```python
from build123d import *

# Parameters (mm, degrees)
SKETCH1_R           = 16.25
BOSS_EXTRUDE1_DEPTH = 84
SKETCH2_R           = 10
BOSS_EXTRUDE2_DEPTH = 3
SKETCH3_R           = 3
BOSS_EXTRUDE3_DEPTH = 17
CUT_EXTRUDE1_DEPTH  = 12
SKETCH5_R           = 16.25
BOSS_EXTRUDE4_DEPTH = 18
SKETCH6_W           = 8.15482979
SKETCH6_H           = 20.288083416
BOSS_EXTRUDE5_DEPTH = 16


with BuildPart() as part:
    # Sketch1 → Boss-Extrude1 (new body)
    with BuildSketch(Plane(origin=(0, 0, 0), x_dir=(0, 0, -1), z_dir=(1, 0, 0))):
        Circle(SKETCH1_R)
    extrude(amount=BOSS_EXTRUDE1_DEPTH)

    # Sketch2 → Boss-Extrude2 (add)
    with BuildSketch(Plane(origin=(84, 0, 0), x_dir=(0, 0, -1), z_dir=(1, 0, 0))):
        Circle(SKETCH2_R)
    extrude(amount=BOSS_EXTRUDE2_DEPTH)

    # Sketch3 → Boss-Extrude3 (add)
    with BuildSketch(Plane(origin=(87, 0, 0), x_dir=(0, 0, -1), z_dir=(1, 0, 0))):
        Circle(SKETCH3_R)
    extrude(amount=BOSS_EXTRUDE3_DEPTH)

    # Sketch4 → Cut-Extrude1 (cut)
    with BuildSketch(Plane(origin=(104, 0, 0), x_dir=(0, 0, -1), z_dir=(1, 0, 0))):
        Polygon((-63.514658307, 2.5), (-1.658312395, 2.5), (1.658312395, 2.5), (63.514658307, 2.5), (63.514658307, 126.212691825), (-63.514658307, 126.212691825), align=None)
    extrude(amount=-CUT_EXTRUDE1_DEPTH, mode=Mode.SUBTRACT)

    # Sketch5 → Boss-Extrude4 (add)
    with BuildSketch(Plane.ZY):
        Circle(SKETCH5_R)
        with BuildLine():
            Line((-16.25, 23.75), (-16.25, 0))
            ThreePointArc((-16.25, 0), (0, 16.25), (16.25, 0))
            Line((16.25, 0), (16.25, 23.75))
            Line((16.25, 23.75), (-16.25, 23.75))
        make_face()
    extrude(amount=BOSS_EXTRUDE4_DEPTH)

    # Sketch6 → Boss-Extrude5 (add)
    with BuildSketch(Plane(origin=(0, 23.75, 0), x_dir=(1, 0, 0), z_dir=(0, 1, 0))):
        with Locations((-9, 0)):
            Rectangle(SKETCH6_W, SKETCH6_H)
    extrude(amount=BOSS_EXTRUDE5_DEPTH)


solid = part.part
```
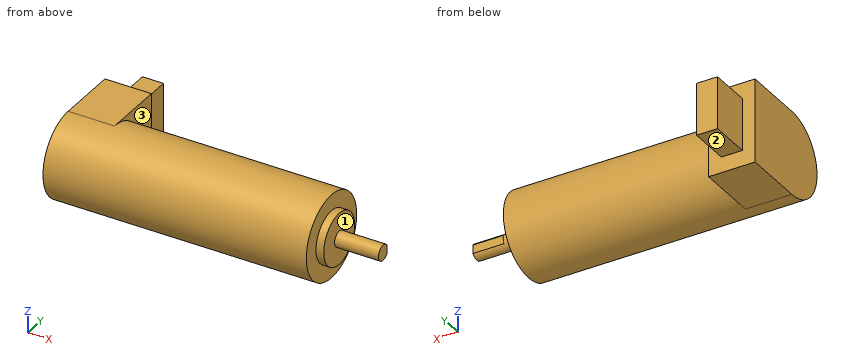
Source: CAD feature listing. Evaluate the final solid. Frame: model axes, mm. Face numbers are marked on the shaded views. A direction names the side the tool comes from. Give positions to 0.01 mm unless a question says otherwise; leave off trailing zeros. Order: outer loops, then holes, each group sorted by start corner. A loop starts at its lowest first (then second) coordinate and runs counter-clockwise, first axis right, second up.
(1) Section query D-D (y = -5). Return the cut outline in (x, z), plus the area to 3 significant figures.
(2) Section query A-A (y = 26). Return the cut outline in (x, z), plus the area to 3 significant figures.
(3) Contact query for flat-ended pins moving along their axis: P1, Ø8, axis at x = 45.5, y = -7.5, coming from the +Z side; P2, Ø10, axis at y = -2, z = 4, coming from the +X side; P3, Ø1.5, axis at x = 73.5, z = 9, coming from the -Y side; P4, Ø8, axis at y = 29.5, z = -2, coming from the +X side. Output: stop coordinate, or through.
(4) Access query for the marked faces 1, 2 and 3. Directions: +Z, -Z, +X, -X, +Y, -Y. A direction counts if a zero-diameter tool reaches every point of the face in a straight line with its end or side. Return the directions, or none.
(5) Material intervals for line 1 along X through (y, z) = (1, 7.5); line 2 along X through (y, z) = (27, 0.5); line 3 along Z through (x, y) = (20, -0.5), sorted ascending.
(6) Section query B-B (z = 6.5). Return the cut outline in (x, y).
(7) Section query C-C (x = 96). Return the cut outline in (y, z).
Outcome:
1. outline: (-18, -15.46) - (84, -15.46) - (84, -8.66) - (87, -8.66) - (87, 8.66) - (84, 8.66) - (84, 15.46) - (-18, 15.46) - close
1. area: 3,210 mm2
2. outline: (-13.08, -10.14) - (-4.92, -10.14) - (-4.92, 10.14) - (-13.08, 10.14) - close
2. area: 165 mm2
3. P1: stops at z = 15.87
3. P2: stops at x = 104
3. P3: stops at y = -14
3. P4: stops at x = -4.92
4. face 1: +X
4. face 2: -Z, +X, -X, +Y
4. face 3: +X, +Y
5. line 1: x = -18 to 87
5. line 2: x = -13.08 to -4.92
5. line 3: z = -16.24 to 16.24
6. outline: (-18, -14.89) - (84, -14.89) - (84, -7.6) - (87, -7.6) - (87, 7.6) - (84, 7.6) - (84, 14.89) - (0, 14.89) - (0, 23.75) - (-4.92, 23.75) - (-4.92, 39.75) - (-13.08, 39.75) - (-13.08, 23.75) - (-18, 23.75) - close
7. outline: (2.5, -1.66) - (2.5, 1.66) arc R3 ccw (long way) to start
